```python
from build123d import *

# Parameters (mm, degrees)
SKETCH1_W           = 101.6
SKETCH1_H           = 76.2
BOSS_EXTRUDE1_DEPTH = 5.85
SKETCH2_W           = 41.475447085
SKETCH2_H           = 25.4
BOSS_EXTRUDE2_DEPTH = 5.85
CAVITY1_START       = -38.1
CAVITY1_OUTLINE_W   = 33.866666667
CAVITY1_OUTLINE_H   = 5.85
CAVITY1_DEPTH       = 11.7
CAVITY1_START_2     = 12.7
CAVITY1_2_OUTLINE_W = 5.85
CAVITY1_2_OUTLINE_H = 5.85
CAVITY1_2_DEPTH     = 25.4
CAVITY1_START_3     = -26.4
CAVITY1_3_OUTLINE_W = 5.85
CAVITY1_3_OUTLINE_H = 5.85
CAVITY1_3_DEPTH     = 13.7


# Read off the part's stored shape, not the designer's step: Cavity1
with BuildPart() as part:
    # Sketch1 → Boss-Extrude1 (new body)
    with BuildSketch(Plane(origin=(0, 0, 0), x_dir=(1, 0, 0), z_dir=(0, 1, 0))):
        Rectangle(SKETCH1_W, SKETCH1_H)
    extrude(amount=BOSS_EXTRUDE1_DEPTH)

    # Sketch2 → Boss-Extrude2 (add)
    with BuildSketch(Plane(origin=(0, 5.85, 0), x_dir=(1, 0, 0), z_dir=(0, 1, 0))):
        with Locations((-1.285396087, -50.8)):
            Rectangle(SKETCH2_W, SKETCH2_H)
    extrude(amount=-BOSS_EXTRUDE2_DEPTH)

    # Cavity1 outline → Cavity1 (cut)
    with BuildSketch(Plane.XY.offset(CAVITY1_START)):
        with Locations((33.866666667, 2.925)):
            Rectangle(CAVITY1_OUTLINE_W, CAVITY1_OUTLINE_H)
        with Locations((-33.866666667, 2.925)):
            Rectangle(CAVITY1_OUTLINE_W, CAVITY1_OUTLINE_H)
    extrude(amount=CAVITY1_DEPTH, mode=Mode.SUBTRACT)

    # Cavity1 2 outline → Cavity1 2 (cut)
    with BuildSketch(Plane.XY.offset(CAVITY1_START_2)):
        with Locations((47.875, 2.925)):
            Rectangle(CAVITY1_2_OUTLINE_W, CAVITY1_2_OUTLINE_H)
        with Locations((-47.875, 2.925)):
            Rectangle(CAVITY1_2_OUTLINE_W, CAVITY1_2_OUTLINE_H)
    extrude(amount=CAVITY1_2_DEPTH, mode=Mode.SUBTRACT)

    # Cavity1 3 outline → Cavity1 3 (cut)
    with BuildSketch(Plane.XY.offset(CAVITY1_START_3)):
        with Locations((47.875, 2.925)):
            Rectangle(CAVITY1_3_OUTLINE_W, CAVITY1_3_OUTLINE_H)
        with Locations((-47.875, 2.925)):
            Rectangle(CAVITY1_3_OUTLINE_W, CAVITY1_3_OUTLINE_H)
    extrude(amount=CAVITY1_3_DEPTH, mode=Mode.SUBTRACT)


solid = part.part
```
Input: part model. Units: mm. Frame: model coordinates. A direction names the side the tool comes from. Give positions to 0.01 mm unless a question says otherwise; leave off trailing zeros. Order: outer loops, then holes, each group sorted by start corner. A loop starts at its lowest first (then second) coordinate and runs counter-clockwise, first axis right, second up. Notation, with made-up numbers: M 42,-1 L 55,-1 A12 cw 55,9 Z; hole C -34,2.5 d6. An arc over 180 degrees is marked long. Return JSON: item names as keys, results as strings.
Item 1: Cut plane B-B (x = -35.5). Return loops of the section in (y, z).
Solutions:
{"outline": "M 0,-26.4 L 5.85,-26.4 L 5.85,38.1 L 0,38.1 Z"}
Item 2: First-contact query: P1, Ø1.8, axis at y = 4, z = 51, coming from the +X side; P2, Ø3, axis at y = 4, z = 27.5, coming from the +X side; P3, Ø1.8, axis at x = -47.5, y = 3, coming from the +Z side; P4, Ø3, axis at x = -25.5, z = 51.5, coming from the -Y side. Flat tips, straight axial feed; report the tip coordinate or a pass-through.
Solutions:
{"P1": "x = 19.45", "P2": "x = 44.95", "P3": "z = 12.7", "P4": "through"}
Item 3: Cut plane C-C (z = -30.5). Return loops of the section in (x, y).
Solutions:
{"outline": "M -16.93,0 L 16.93,0 L 16.93,5.85 L -16.93,5.85 Z"}
Item 4: Cut plane A-A (y = 3.6). Return loops of the section in (x, z).
Solutions:
{"outline": "M -50.8,-12.7 L -44.95,-12.7 L -44.95,-26.4 L -16.93,-26.4 L -16.93,-38.1 L 16.93,-38.1 L 16.93,-26.4 L 44.95,-26.4 L 44.95,-12.7 L 50.8,-12.7 L 50.8,12.7 L 44.95,12.7 L 44.95,38.1 L 19.45,38.1 L 19.45,63.5 L -22.02,63.5 L -22.02,38.1 L -44.95,38.1 L -44.95,12.7 L -50.8,12.7 Z"}
Item 5: Access query for faces 1 (the flat face through (44.95, 3, 25)), 2 (the flat face through (-44.95, 3, 25)), 3 (the flat face through (-48, 3, -12.7)). Directions: +Z, -Z, +X, -X, +Y, -Y. A direction counts if a zero-diameter tool reaches every point of the face in a straight line with its end or side. Return the directions, or none.
Solutions:
{"face 1": "+Z, +X, +Y, -Y", "face 2": "+Z, -X, +Y, -Y", "face 3": "-Z, -X, +Y, -Y"}
Item 6: Ray query, probe 1 along X at (y, z) = (2.05, -23.5); probe 2 along Z at (x, y) = (26.5, 1.35); probe 3 along X at (y, z) = (5.25, 45.5). Return the intervals inside material, ascending.
Solutions:
{"probe 1": "-44.95 to 44.95", "probe 2": "-26.4 to 38.1", "probe 3": "-22.02 to 19.45"}
